from build123d import *

# Parameters (mm, degrees)
SKETCH2_R           = 1.5
BOSS_EXTRUDE1_DEPTH = 6.35
FILLET1_R           = 1.27
FILLET2_R           = 2.54
FILLET3_R           = 6.35
FILLET4_R           = 2.54


with BuildPart() as part:
    # Sketch2 → Boss-Extrude1 (new body)
    with BuildSketch(Plane(origin=(0, 0, 0), x_dir=(1, 0, 0), z_dir=(0, 1, 0))):
        Polygon((-2.553535433, -69.492861925), (-4.46233448, -82.048597116), (-1.323400683, -82.525796878), (-0.369001159, -76.247929282), (12.186734033, -78.15672833), (12.663933794, -75.017794532), (14.668172794, -61.834272581), (11.529238997, -61.357072819), (10.002199758, -71.401660972), align=None)
        with Locations(Location((9.524999997, -74.54059477, 0), (0, 0, 270))):
            Circle(SKETCH2_R, mode=Mode.SUBTRACT)
    extrude(amount=BOSS_EXTRUDE1_DEPTH)

    # Fillet1
    fillet1_edges = [part.edges().sort_by_distance(p)[0] for p in [
        (-0.369001159, 3.175, 76.247929282),
        (-1.323400683, 3.175, 82.525796878),
    ]]
    fillet(fillet1_edges, radius=FILLET1_R)

    # Fillet2
    fillet2_edges = [part.edges().sort_by_distance(p)[0] for p in [
        (11.529238997, 3.175, 61.357072819),
    ]]
    fillet(fillet2_edges, radius=FILLET2_R)

    # Fillet3
    fillet3_edges = [part.edges().sort_by_distance(p)[0] for p in [
        (-2.553535433, 3.175, 69.492861925),
    ]]
    fillet(fillet3_edges, radius=FILLET3_R)

    # Fillet4
    fillet4_edges = [part.edges().sort_by_distance(p)[0] for p in [
        (12.186734033, 3.175, 78.15672833),
    ]]
    fillet(fillet4_edges, radius=FILLET4_R)


solid = part.part
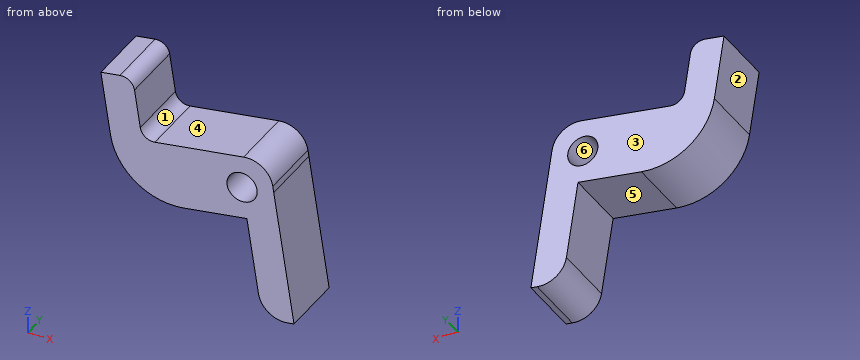
Geometry: final body of the model. Coordinates: model frame, mm. Face numbers are marked on the shaded views. A direction names the side the tool comes from. Give positions to 0.01 mm unless a question says otherwise; leave off trailing zeros. Loops run counter-clockwise (first coordinate to the right, second up) from the corner with the lowest first, then second, coordinate; pieces in that order, holes last. Notation, with made-up numbers: (36, -13) - (53, -13) arc R18 ccw to (53, -8) - close; hole circle Ø7 at (45.5, 57.5). An arc over 180 degrees is marked (long way). Answer as CSV lines item,"result". Start each with the question number.
1. Draft query along X for the marked faces 1, 2 and 3. Return one class per face: released by +X, released by -X, zero draft, split by the parting line, or undercut.
2. Ray query, L1, parallel to X at y = 5.75, z = 73.5; L2, parallel to Z at x = 0.25, y = 1; L3, parallel to X at y = 3, z = 72. Return the intervals inside material, ascending.
3. Section A-A, the plane x = 9. Return loops of the section in (y, z).
4. Section D-D, the plane x = -3. Return loops of the section in (y, z), plus the area to 3 significant figures.
5. Reachability of the marked faces 4, 5 and 6 from +Z, -Z, +X, -X, +Y, -Y: full face, straight path, thin tool, end or side. Return the list, or none.
6. Section C-C, the plane z = 69.75. Return loops of the section in (x, y), plus the area to 3 significant figures.
7. Pin query (flat end, axial travel): P1, Ø1.5, axis at y = 4.5, z = 71, coming from the -X side; P2, Ø3, axis at y = 4.5, z = 68.5, coming from the -X side; P3, Ø1, axis at y = 5, z = 70, coming from the +X side; P4, Ø1.5, axis at x = 11, z = 79, coming from the -Y side. Return the tip coordinate at first contact, or that it passes through.
Answers:
1,face 1,"undercut"
1,face 2,"released by -X"
1,face 3,"zero draft"
2,L1,"x = -2.7 to 8.44, 10.61 to 12.89"
2,L2,"z = 70.9 to 76.51"
2,L3,"x = -1.47 to 13.12"
3,outline,"(0, 71.25) - (6.35, 71.25) - (6.35, 73.14) - (0, 73.14) - close; (0, 75.95) - (6.35, 75.95) - (6.35, 77.67) - (0, 77.67) - close"
4,outline,"(0, 74.07) - (6.35, 74.07) - (6.35, 82.27) - (0, 82.27) - close"
4,area,"52.1 mm2"
5,face 4,"+Z, +Y, -Y"
5,face 5,"-Z, +Y, -Y"
5,face 6,"+Y, -Y"
6,outline,"(10.25, 0) - (13.46, 0) - (13.46, 6.35) - (10.25, 6.35) - close"
6,area,"20.4 mm2"
7,P1,"stops at x = -1.18"
7,P2,"stops at x = 10.22"
7,P3,"stops at x = 13.5"
7,P4,"passes through"
